Part model, mm, in its own coordinate system. A direction names the side the tool comes from. Coordinates: 2 decimals unless noted, no trailing zeros. Loops run counter-clockwise (first coordinate to the right, second up) from the corner with the lowest first, then second, coordinate; pieces in that order, holes last. Notation, with made-up numbers: (-5, -3) - (51, -3) arc R24 cw to (51, 7) - close; hole circle Ø6 at (-37, -13.5). An arc over 180 degrees is marked (long way). Use a Markdown table: item, result. Add a question column.
1. 3-axis set-ups, long thin cutter, end or side, ignore diameter. For faces 4 (the flat face through (19, -0.343, -10)), 5 (the flat face through (2, 5, -10)), 6 (the flat face through (35, 4, -1)): which of +Z, -Z, +X, -X, +Y, -Y reach the whole face in a straight line?
2. Band-saw the part on D-D, the plane z = -10.25. Give the cut face in (x, y).
3. Pull direction Z, two halves, no side cores. Call faces 1 (the flat face through (34.986, 4.727, -10.765)), 2 (the flat face through (17, 5, -5.751)), 3 (the flat face through (18, 5, 8.649)): pulls with the +Z half, pulls with the -Z half, needs draft (parallel to the pull), parting line crosses it, or undercut.
4. Drop flat-ended pins along their axis: pin 1 (6 mm diameter, centred on x = 15, z = -7, fed in from +Y); pin 2 (1.5 mm diameter, centred on x = 20, z = -7.5, fed in from -Y); pin 3 (2 mm diameter, centred on y = 3, z = -8.5, fed in from +X). Give the stop position or say it passes through.
5. Band-saw the part on C-C, the plane y = -1. Give the cut face in (x, z).
6. Band-saw the part on A-A, the plane x = 3. Give the cut face in (y, z).
7. Band-saw the part on B-B, the plane y = 3. Give the cut face in (x, z).
8. Wall check: probe 1 along Z at (x, y) = (5, 4); probe 2 along Y at (x, z) = (3, 0.75); probe 3 along X at (y, z) = (14, 0). Give the ranges that are in metal, low to high. Write a range as [from, to].
from build123d import *

# Parameters (mm, degrees)
F1_DEPTH    = 35
F2_T        = 2
F3_T1_DEPTH = 14
F3_T4_ANGLE = 180
F3_T6_ANGLE = 180
F4_R        = 1
F5_DEPTH    = 3
F6_W        = 1
F6_H        = 10
F6_W_2      = 33
F7_DEPTH    = 4
F8_SIZE     = 2


# Not quite as in the source:
# - a fillet or chamfer that OpenCascade refuses, or shapes differently, is made with other operations: its cross-section is extruded or revolved along the edge and cut away or added


with BuildPart() as f1:
    # F0 (on Right) → F1 (new body)
    with BuildSketch(Plane.YZ):
        with BuildLine():
            ThreePointArc((-8.5429217076, 0.448732347), (-6.726983751, -3.9353296963), (-2.3429217076, -5.751267653))
            Line((-2.3429217076, -5.751267653), (11.6570782924, -5.751267653))
            ThreePointArc((11.6570782924, -5.751267653), (16.0411403357, -3.9353296963), (17.8570782924, 0.448732347))
            ThreePointArc((17.8570782924, 0.448732347), (16.0411403357, 4.8327943904), (11.6570782924, 6.648732347))
            Line((11.6570782924, 6.648732347), (-2.3429217076, 6.648732347))
            ThreePointArc((-2.3429217076, 6.648732347), (-6.726983751, 4.8327943904), (-8.5429217076, 0.448732347))
        make_face()
    extrude(amount=F1_DEPTH)

    # F2
    f2_openings = [f1.faces().sort_by_distance(p)[0] for p in [
        (0, 4.657078, 0.448732),
    ]]
    offset(amount=F2_T, openings=f2_openings, kind=Kind.INTERSECTION)

    # F3: chamfer of 1 on 4 edges, made by hand

    # F3_s2 → F3_t1 (cut)
    with BuildSketch(Plane.XZ.offset(-11.6570782924)):
        Polygon((37, -6.751267653), (36, -7.751267653), (37, -7.751267653), align=None)
        Polygon((37, 7.648732347), (36, 8.648732347), (37, 8.648732347), align=None)
    extrude(amount=F3_T1_DEPTH, mode=Mode.SUBTRACT)

    # F3_s3 → F3_t4 (revolve, cut)
    with BuildSketch(Plane.XZ.offset(2.3429217076)):
        Polygon((36, -7.751267653), (37, -6.751267653), (37, -7.751267653), align=None)
    revolve(axis=Axis((37, -2.3429217076, 0.448732347), (-1, 0, 0)), revolution_arc=F3_T4_ANGLE, mode=Mode.SUBTRACT)

    # F3_s5 → F3_t6 (revolve, cut)
    with BuildSketch(Plane.XZ.offset(-11.6570782924)):
        Polygon((37, 7.648732347), (36, 8.648732347), (37, 8.648732347), align=None)
    revolve(axis=Axis((37, 11.6570782924, 0.448732347), (-1, 0, 0)), revolution_arc=F3_T6_ANGLE, mode=Mode.SUBTRACT)

    # F4 (on face) → F5 (cut)
    with BuildSketch(Plane.YZ.offset(37)):
        with Locations((4.6570782924, 0.448732347)):
            Circle(F4_R)
    extrude(amount=-F5_DEPTH, mode=Mode.SUBTRACT)

    # F6 (on face) → F7 (join)
    with BuildSketch(Plane(origin=(0, 0, -7.751267653), x_dir=(1, 0, 0), z_dir=(0, 0, -1))):
        with Locations((35.5, -4.6570782924)):
            Rectangle(F6_W, F6_H)
        with Locations((18.5, -4.6570782924)):
            Rectangle(F6_W_2, F6_H)
    extrude(amount=F7_DEPTH)

    # F8
    f8_edges = [f1.edges().sort_by_distance(p)[0] for p in [
        (36, 4.657078, -11.751268),
    ]]
    chamfer(f8_edges, length=F8_SIZE)


solid = f1.part
Geometry check:
| question | item | result |
|---|---|---|
| 1 | face 4 | -Z, +X, -X, -Y |
| 1 | face 5 | -Z, -X, +Y, -Y |
| 1 | face 6 | -X |
| 2 | outline | (2, -0.34) - (35.5, -0.34) - (35.5, 9.66) - (2, 9.66) - close |
| 3 | face 1 | pulls with the -Z half |
| 3 | face 2 | undercut |
| 3 | face 3 | pulls with the +Z half |
| 4 | pin 1 | stops at y = 18.55 |
| 4 | pin 2 | stops at y = -6.27 |
| 4 | pin 3 | stops at x = 36.25 |
| 5 | outline | (0, -7.75) - (36, -7.75) - (37, -6.75) - (37, 7.65) - (36, 8.65) - (0, 8.65) - (0, 6.65) - (35, 6.65) - (35, -5.75) - (0, -5.75) - close |
| 6 | outline | (-2.34, -7.75) - (-0.34, -7.75) - (-0.34, -11.75) - (9.66, -11.75) - (9.66, -7.75) - (11.66, -7.75) arc R8.2 ccw to (11.66, 8.65) - (-2.34, 8.65) arc R8.2 ccw to start; hole (-2.34, -5.75) - (11.66, -5.75) arc R6.2 ccw to (11.66, 6.65) - (-2.34, 6.65) arc R6.2 ccw to start |
| 7 | outline | (0, -7.75) - (2, -7.75) - (2, -11.75) - (34, -11.75) - (36, -9.75) - (36, -7.75) - (37, -6.75) - (37, 7.65) - (36, 8.65) - (0, 8.65) - (0, 6.65) - (35, 6.65) - (35, -5.75) - (0, -5.75) - close |
| 8 | probe 1 | z = [-11.75, -5.75], [6.65, 8.65] |
| 8 | probe 2 | y = [-10.54, -8.54], [17.85, 19.85] |
| 8 | probe 3 | x = [35, 37] |
